Input: dimensioned drawing with shaded views. Units: mm. Origin: part minimum x, y, z. Round coordinates to 2 decimals unless told otherwise and drop trailing zeros. Loops run counter-clockwise (first coordinate to the right, second up) from the corner with the lowest first, then second, coordinate; pieces in that order, holes last. Notation, with made-up numbers: (27, 28) - (52, 28) arc R26 cw to (52, 59) - close; hole circle Ø7 at (29, -18.75). An arc over 180 degrees is marked (long way). Write each question's results on one line, items separated by ' | '.
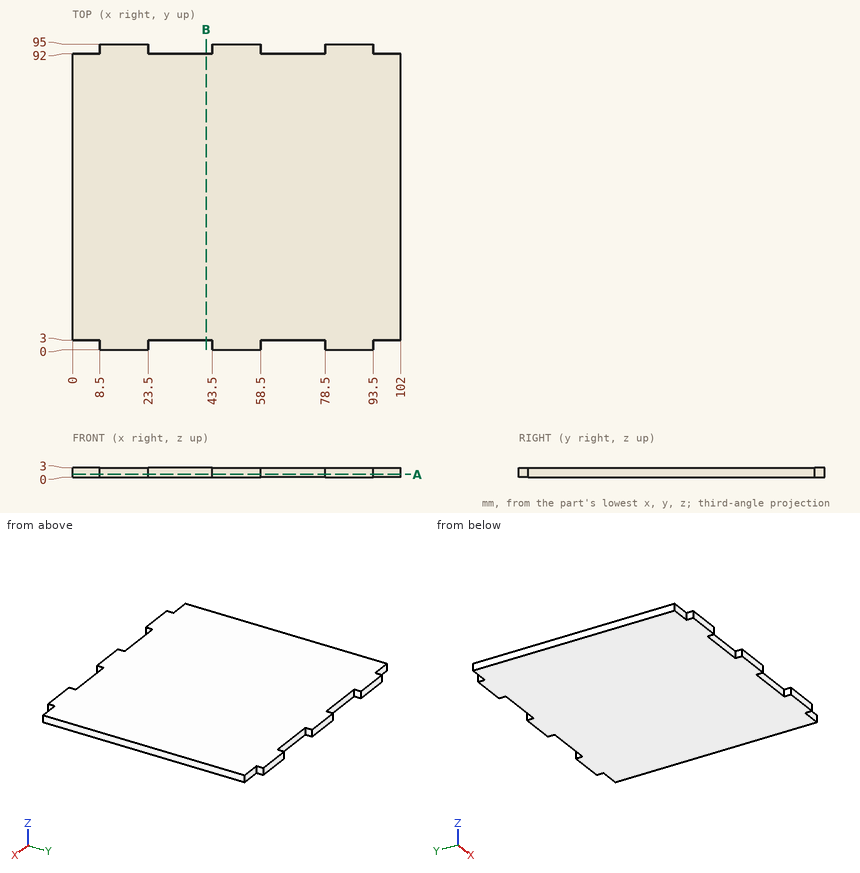
1. Line query: line 1 (Y direction, x = 60, z = 2.2). Output: solid intervals per line, ascending. Write a range as [from, to].
Answer:
line 1: [3, 92]
2. Section query A-A, the plane z = 0.9. Output: boundary loops of the cut face in (x, y).
Answer:
outline: (0, 3) - (8.5, 3) - (8.5, 0) - (23.5, 0) - (23.5, 3) - (43.5, 3) - (43.5, 0) - (58.5, 0) - (58.5, 3) - (78.5, 3) - (78.5, 0) - (93.5, 0) - (93.5, 3) - (102, 3) - (102, 92) - (93.5, 92) - (93.5, 95) - (78.5, 95) - (78.5, 92) - (58.5, 92) - (58.5, 95) - (43.5, 95) - (43.5, 92) - (23.5, 92) - (23.5, 95) - (8.5, 95) - (8.5, 92) - (0, 92) - close
3. Contact query for flat-ended pins moving along their axis: pin 1 (1.5 mm diameter, centred on x = 41.5, z = 2, fed in from -Y); pin 2 (1.5 mm diameter, centred on y = 1.5, z = 1, fed in from +X); pin 3 (1.5 mm diameter, centred on x = 98, z = 2, fed in from +Y). Output: stop coordinate, or through.
Answer:
pin 1: y = 3 | pin 2: x = 93.5 | pin 3: y = 92
4. Section query B-B, the plane x = 41.5. Output: boundary loops of the cut face in (y, z).
Answer:
outline: (3, 0) - (92, 0) - (92, 3) - (3, 3) - close
